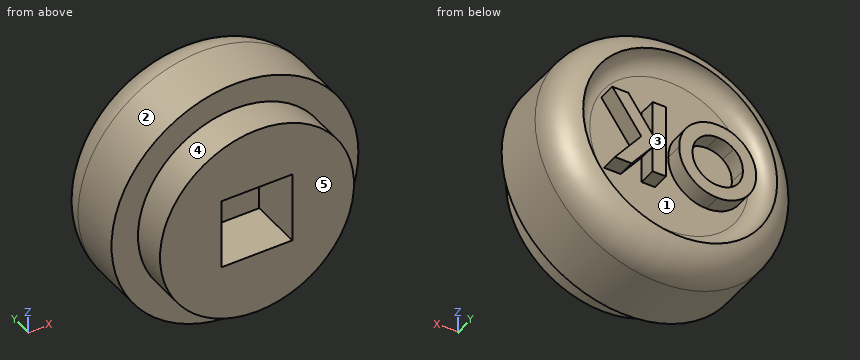
from build123d import *

# Parameters (mm, degrees)
SKETCH_1_R          = 5.5
EXTRUDE_1_DEPTH     = 7
CUT_EXTRUDE_START   = -1
SKETCH_2_R          = 5.5
CUT_EXTRUDE_1_DEPTH = 1
EXTRUDE_2_DEPTH     = 1
SKETCH_5_W          = 4
SKETCH_5_H          = 4
CUT_EXTRUDE_2_DEPTH = 3
FILLET_3_R          = 1


with BuildPart() as part:
    # Эскиз1 → Бобышка-Вытянуть1 (new body)
    with BuildSketch(Plane(origin=(0, 0, 0), x_dir=(1, 0, 0), z_dir=(0, 1, 0))):
        with Locations(Location((0, 0, 0), (0, 0, 270))):
            Circle(SKETCH_1_R)
    extrude(amount=EXTRUDE_1_DEPTH)

    # Эскиз6 → Повернуть3 (revolve)
    with BuildSketch(Plane.XY, mode=Mode.PRIVATE) as revolve_3_sk:
        with BuildLine():
            Line((-4.665230635, 2), (-7, 2))
            Line((-7, 2), (-7, 3))
            Line((-7, 3), (-7, 5.035898385))
            ThreePointArc((-7, 5.035898385), (-6.582112259, 6.271585962), (-5.5, 7))
            Line((-5.5, 7), (-4.665230635, 7))
            Line((-4.665230635, 7), (-4.665230635, 3))
            Line((-4.665230635, 3), (-4.665230635, 2))
        make_face()
    revolve(revolve_3_sk.sketch.rotate(Axis((0, -1000, 0), (0, 1, 0)), 180), axis=Axis((0, -1000, 0), (0, 1, 0)))

    # Эскиз2 → Вырез-Вытянуть1 (cut)
    with BuildSketch(Plane(origin=(0, 7, 0), x_dir=(1, 0, 0), z_dir=(0, 1, 0)).offset(CUT_EXTRUDE_START)):
        with Locations(Location((0, 0, 0), (0, 0, 180))):
            Circle(SKETCH_2_R)
    extrude(amount=CUT_EXTRUDE_1_DEPTH, mode=Mode.SUBTRACT)

    # Эскиз3 → Бобышка-Вытянуть2 (add)
    # profile 1 of 2: a face of its own
    with BuildSketch(Plane(origin=(0, 6, 0), x_dir=(1, 0, 0), z_dir=(0, 1, 0))):
        with BuildLine():
            add(Edge.make_bspline(
                [(-2.119769226, 2.297656666), (-2.046747078, 2.295765991), (-1.90258482, 2.292033372), (-1.690574161, 2.26091908), (-1.486262691, 2.2102228), (-1.289742798, 2.139751305), (-1.101506546, 2.047595868), (-0.920889962, 1.936369156), (-0.748540006, 1.803971831), (-0.586222783, 1.653492505), (-0.436212395, 1.489852809), (-0.306228306, 1.313665584), (-0.195382643, 1.129496016), (-0.103513461, 0.936850619), (-0.03353798, 0.734395232), (0.01556671, 0.523162109), (0.04711404, 0.303211345), (0.050742469, 0.153454853), (0.052586544, 0.077344166)],
                knots=[0, 0, 0, 0, 1.014329547, 2.002516266, 2.970391464, 3.935626869, 4.897733899, 5.877609409, 6.878433252, 7.912639331, 8.949961323, 9.958554974, 10.949718813, 11.932905612, 12.9188844, 13.919928257, 14.942845884, 16, 16, 16, 16], degree=3))
            add(Edge.make_bspline(
                [(0.052586544, 0.077344166), (0.050622684, 0.002091069), (0.046752835, -0.146197571), (0.01685461, -0.364121403), (-0.033077009, -0.573091779), (-0.101865651, -0.773581708), (-0.192068673, -0.964620087), (-0.300752725, -1.147426668), (-0.430785771, -1.320304963), (-0.577424997, -1.483162198), (-0.738862058, -1.630990084), (-0.909849534, -1.761263154), (-1.08959791, -1.871651637), (-1.277844091, -1.96210497), (-1.474991763, -2.032302471), (-1.680553946, -2.081831908), (-1.894517921, -2.111931947), (-2.040023801, -2.115776519), (-2.113879803, -2.11772795)],
                knots=[0, 0, 0, 0, 1.051557043, 2.072126891, 3.067553643, 4.050577992, 5.02905126, 6.015227836, 7.017913613, 8.04756643, 9.074058332, 10.072836633, 11.047628519, 12.017157415, 12.98668631, 13.966869689, 14.968021931, 16, 16, 16, 16], degree=3))
            add(Edge.make_bspline(
                [(-2.113879803, -2.11772795), (-2.191124325, -2.11597742), (-2.342899253, -2.112537868), (-2.565022539, -2.079829301), (-2.777835841, -2.030558773), (-2.979551403, -1.957025153), (-3.172223527, -1.865101945), (-3.354436593, -1.751893002), (-3.526129367, -1.617585413), (-3.68631699, -1.465618843), (-3.831447364, -1.299334085), (-3.959553386, -1.123668983), (-4.067613658, -0.939965466), (-4.155632133, -0.748137555), (-4.225022363, -0.549377415), (-4.273969286, -0.342474539), (-4.302883401, -0.127925156), (-4.30691097, 0.017801074), (-4.308951918, 0.09164705)],
                knots=[0, 0, 0, 0, 1.067978421, 2.098431617, 3.099715153, 4.085208694, 5.062210972, 6.048429807, 7.046490867, 8.072918869, 9.098532598, 10.095778865, 11.076610158, 12.041847152, 13.011192615, 13.984257998, 14.978533688, 16, 16, 16, 16], degree=3))
            add(Edge.make_bspline(
                [(-4.308951918, 0.09164705), (-4.308311351, 0.141326757), (-4.307038327, 0.240057111), (-4.291703421, 0.386370456), (-4.269625564, 0.529827961), (-4.236973461, 0.669857659), (-4.197309501, 0.807447394), (-4.145919239, 0.941316447), (-4.087423212, 1.072894908), (-4.019076113, 1.200628669), (-3.943080748, 1.323342475), (-3.860163038, 1.440457461), (-3.770114489, 1.550557538), (-3.673225176, 1.654366237), (-3.569161205, 1.751201216), (-3.459291432, 1.842433309), (-3.341485021, 1.925639068), (-3.218320386, 2.002850542), (-3.0904919, 2.072671539), (-2.958519942, 2.132101084), (-2.825123394, 2.183999893), (-2.688520259, 2.224960728), (-2.550174481, 2.2583229), (-2.408608118, 2.280385876), (-2.265100139, 2.295720358), (-2.16832783, 2.297009698), (-2.119769226, 2.297656666)],
                knots=[0, 0, 0, 0, 1.034744296, 2.056386356, 3.06226378, 4.057406941, 5.050368692, 6.043467995, 7.042652155, 8.049140477, 9.059438543, 10.048523776, 11.036952808, 12.020949711, 13.004946614, 13.997082645, 14.994316842, 16.007702937, 17.024872941, 18.026463647, 19.021641123, 20.005082605, 20.995858141, 21.984425357, 22.988620895, 24, 24, 24, 24], degree=3))
        make_face()
        with BuildLine():
            add(Edge.make_bspline(
                [(-2.131548072, 1.543810512), (-2.180691967, 1.542491871), (-2.277682351, 1.539889401), (-2.419949581, 1.520062101), (-2.556531146, 1.48839565), (-2.686669921, 1.442527182), (-2.810929937, 1.384148264), (-2.92953147, 1.313462878), (-3.040832134, 1.228041294), (-3.146316015, 1.132469416), (-3.241603344, 1.02598038), (-3.325792705, 0.911859268), (-3.39624564, 0.790296659), (-3.455250415, 0.662421843), (-3.499667933, 0.5267969), (-3.531305199, 0.384484194), (-3.55129877, 0.235238516), (-3.553818985, 0.133497931), (-3.555105764, 0.081550896)],
                knots=[0, 0, 0, 0, 1.033739768, 2.040188636, 3.016340934, 3.979330865, 4.937572243, 5.900995986, 6.878200029, 7.884839167, 8.891893314, 9.879764717, 10.863503415, 11.843163062, 12.837761627, 13.859916423, 14.907309254, 16, 16, 16, 16], degree=3))
            add(Edge.make_bspline(
                [(-3.555105764, 0.081550896), (-3.553399691, 0.023981897), (-3.550056071, -0.088843804), (-3.526529955, -0.253430896), (-3.48627911, -0.408867069), (-3.428157674, -0.554392109), (-3.356071845, -0.691621961), (-3.266552686, -0.818874678), (-3.161049983, -0.936912192), (-3.079771556, -1.005827408), (-3.038519226, -1.040804873)],
                knots=[0, 0, 0, 0, 1.078454662, 2.113592447, 3.107694534, 4.079536787, 5.043276885, 6.005368276, 6.987637804, 8, 8, 8, 8], degree=3))
            add(Edge.make_bspline(
                [(-3.038519226, -1.040804873), (-3.004725691, -1.06664488), (-2.937899997, -1.117742715), (-2.83123164, -1.183235073), (-2.721384236, -1.239368557), (-2.607528848, -1.284723748), (-2.489905935, -1.320399379), (-2.368531624, -1.345382437), (-2.243577894, -1.361061466), (-2.159078326, -1.362935407), (-2.116403841, -1.363881796)],
                knots=[0, 0, 0, 0, 1.023928204, 2.024787132, 3.009472467, 3.9914905, 4.972207045, 5.96565515, 6.972602802, 8, 8, 8, 8], degree=3))
            add(Edge.make_bspline(
                [(-2.116403841, -1.363881796), (-2.068104976, -1.362551974), (-1.97307544, -1.359935508), (-1.833456591, -1.340352294), (-1.699697494, -1.307210424), (-1.570967759, -1.26174433), (-1.447638587, -1.202632414), (-1.330312721, -1.12975459), (-1.218784456, -1.044005703), (-1.11343496, -0.947178757), (-1.01714054, -0.840270228), (-0.933126865, -0.725540405), (-0.860433879, -0.60551713), (-0.802656109, -0.478501656), (-0.756483756, -0.345692949), (-0.725227261, -0.206502827), (-0.705064789, -0.061505087), (-0.702543864, 0.037171), (-0.70125961, 0.087440319)],
                knots=[0, 0, 0, 0, 1.026359118, 2.019393844, 2.989460624, 3.950973911, 4.916101784, 5.890408035, 6.881132271, 7.902007068, 8.92769091, 9.933912415, 10.920395702, 11.90457117, 12.894218921, 13.903490204, 14.931958862, 16, 16, 16, 16], degree=3))
            add(Edge.make_bspline(
                [(-0.70125961, 0.087440319), (-0.7025883, 0.137420576), (-0.705203622, 0.235799089), (-0.724821305, 0.380424042), (-0.757752997, 0.518999679), (-0.803355621, 0.651752311), (-0.861587756, 0.778812083), (-0.933597699, 0.899732178), (-1.019132775, 1.014395696), (-1.1162244, 1.12202125), (-1.221902667, 1.22092224), (-1.335358845, 1.30675032), (-1.453418304, 1.381332193), (-1.578789904, 1.439756621), (-1.708908647, 1.486303239), (-1.844568523, 1.520580836), (-1.986283354, 1.539750113), (-2.082694884, 1.542444981), (-2.131548072, 1.543810512)],
                knots=[0, 0, 0, 0, 1.055025985, 2.07665775, 3.074803781, 4.057872707, 5.035505728, 6.020516407, 7.023567878, 8.050795229, 9.077271434, 10.074415901, 11.050397877, 12.019801805, 12.988065821, 13.964604439, 14.968634123, 16, 16, 16, 16], degree=3))
        make_face(mode=Mode.SUBTRACT)
    # profile 2 of 2: a face of its own
    with BuildSketch(Plane(origin=(0, 6, 0), x_dir=(1, 0, 0), z_dir=(0, 1, 0))):
        Polygon((0.806432697, 2.189964358), (1.560278851, 2.189964358), (1.560278851, 0.711719166), (2.751625005, 2.189964358), (3.703187505, 2.189964358), (2.206432697, 0.33227205), (3.84874039, -2.010035642), (2.94092789, -2.010035642), (1.560278851, -0.040444296), (1.560278851, -2.010035642), (0.806432697, -2.010035642), align=None)
    extrude(amount=EXTRUDE_2_DEPTH)

    # Эскиз5 → Вырез-Вытянуть2 (cut)
    with BuildSketch(Plane.XZ):
        Rectangle(SKETCH_5_W, SKETCH_5_H)
    extrude(amount=-CUT_EXTRUDE_2_DEPTH, mode=Mode.SUBTRACT)

    # Скругление3
    fillet_3_edges = [part.edges().sort_by_distance(p)[0] for p in [
        (5.5, 6, 0),
    ]]
    fillet(fillet_3_edges, radius=FILLET_3_R - 0.0001)  # a hair under: the kernel refuses the full size


solid = part.part
Work out the finished part from the listing and answer in its coordinate system (mm). Face numbers are marked on the shaded views. A direction names the side the tool comes from. Coordinates: 2 decimals unless noted, no trailing zeros. Loops run counter-clockwise (first coordinate to the right, second up) from the corner with the lowest first, then second, coordinate; pieces in that order, holes last. Notation, with made-up numbers: M -36.5,-40 L -28.5,-40 A25 cw -28.5,-16 Z; hole C 34,33 d11. An arc over 180 degrees is marked long. Answer in a Markdown table with one row per item. Add a question column.
1. A tool of negligible diameter and unlimited length cuts with its end or side. For the marked faces 4 and 5, from which of +Z, -Z, +X, -X, +Y, -Y can it reach the whole face along a straight path? Write none if from no direction.
2. Flat-ended cylindrical pins translate along their axes: P1, Ø0.9, axis at y = 1.5, z = 0, coming from the -X side; P2, Ø0.9, axis at y = 1, z = -1, coming from the +X side; P3, Ø1.5, axis at x = -0.5, y = 3, coming from the +Z side; P4, Ø0.8, axis at y = 6.5, z = 1, coming from the +X side. Find the tip coordinate at first contact, or state that the pin passes through.
3. The mould has two halves that part along Z. Classify the marked faces 1, 2 and 3: pulls with the +Z half, pulls with the -Z half, needs draft (parallel to the pull), parting line crosses it, or undercut.
4. Find section A-A, the plane y = 0.75. Write down the section's boundary in (x, z).
5. Consider L1, parallel to Y at x = -0.25, z = 0.5; L2, parallel to Y at x = 4, z = -0.5; L3, parallel to X at y = 1.75, z = 1.5. Determine where each line is inside the solid, lowest interval first.
6. Find section B-B, the plane y = 3.75. Write down the section's boundary in (x, z), then the cut area to 3 significant figures.
Reported:
| question | item | result |
|---|---|---|
| 1 | face 4 | -Y |
| 1 | face 5 | +Z, -Z, +X, -X, -Y |
| 2 | P1 | stops at x = -5.5 |
| 2 | P2 | stops at x = 5.47 |
| 2 | P3 | stops at z = 7 |
| 2 | P4 | stops at x = 6.63 |
| 3 | face 1 | undercut |
| 3 | face 2 | parting line crosses it |
| 3 | face 3 | needs draft |
| 4 | outline | C 0,0 d11; hole M -2,-2 L 2,-2 L 2,2 L -2,2 Z |
| 5 | L1 | y = 3 to 7 |
| 5 | L2 | y = 0 to 6 |
| 5 | L3 | x = -5.29 to -2, 2 to 5.29 |
| 6 | outline | C 0,0 d14 |
| 6 | area | 154 mm^2 |
